Design review of the part shown in the three views and the two pictorial views. Dimensions are in mm from the part's minimum x, y and z. A direction names the side the tool comes from. Coordinates: 2 decimals unless noted, no trailing zeros. Write each loop counter-clockwise with the first axis right and the second up, starting at its lowest first coordinate (ties: lowest second). Pieces come first, ordered by that corner, then holes. Notation, with made-up numbers: (-2.75, -11) - (41.25, -11) arc R22 cw to (41.25, 18) - close; hole circle Ø11 at (32.5, 82.5). An arc over 180 degrees is marked (long way). Return JSON: item names as keys, results as strings. Group by question number.
(1) We need section A-A on x = 4.5. State the section outline as (y, z) points.
(2) We need section C-C on z = 6. State the section outline as (x, y) points.
(3) To check wall thickness, follow L1, parallel to Y at x = 4.5, z = 5; L2, parallel to Y at x = 6, z = 1; L3, parallel to X at y = 5.75, z = 10.75. State the ranges of each line that lie inside material, in increasing order. Write a range as from..to.
(4) Tool access review of the marked faces 4 and 5: name each direction out of +Z, -Z, +X, -X, +Y, -Y from which nothing blocks a thin tool from reaching the whole face with its end or side.
(5) We need section D-D on x = 1.5. State the section outline as (y, z) points.
(6) Draft analysis for pull direction Y (two halves, no side actions). For the marked faces 1, 2 and 3, state which applies: released by +Y, released by -Y, zero draft, split by the parting line, or undercut.
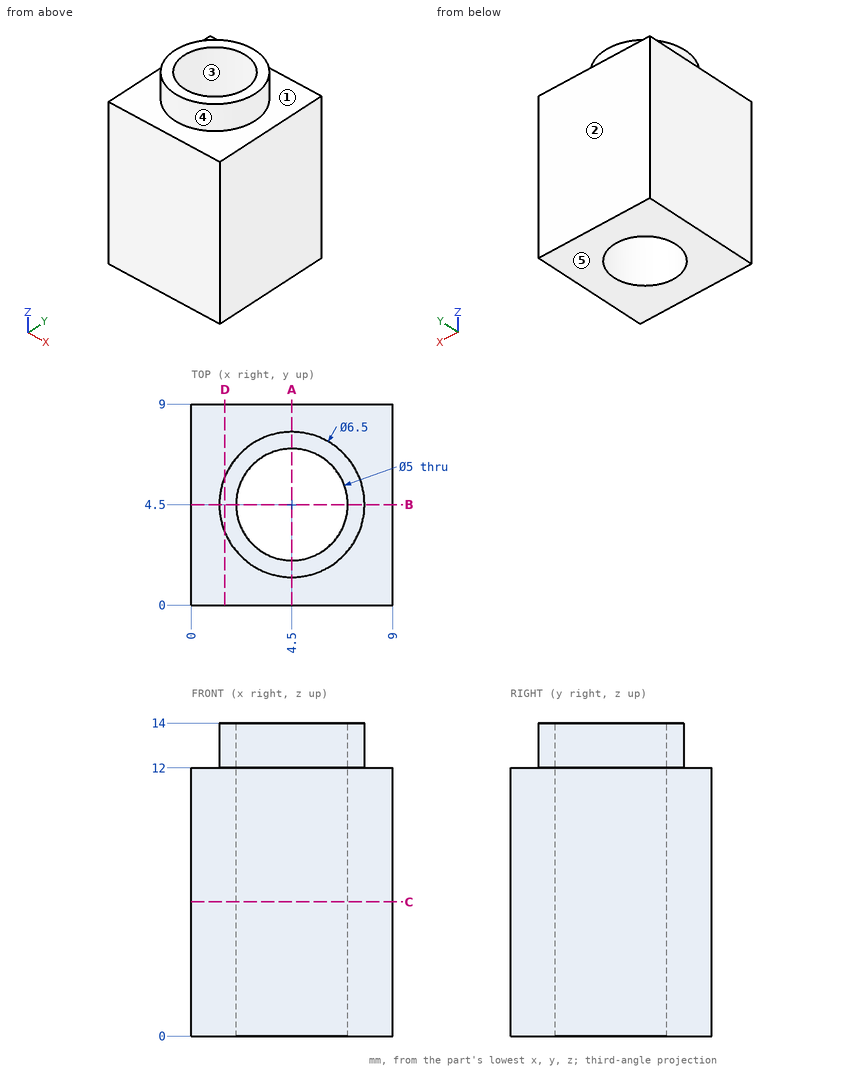
Ans:
{
 "1": {"outline": "(0, 0) - (2, 0) - (2, 14) - (1.25, 14) - (1.25, 12) - (0, 12) - close; (7, 0) - (9, 0) - (9, 12) - (7.75, 12) - (7.75, 14) - (7, 14) - close"},
 "2": {"outline": "(0, 0) - (9, 0) - (9, 9) - (0, 9) - close; hole circle Ø5 at (4.5, 4.5)"},
 "3": {"L1": "0..2, 7..9", "L2": "0..2.5, 6.5..9", "L3": "0..2.33, 6.67..9"},
 "4": {"face 4": "+Z", "face 5": "-Z, +X, -X, +Y, -Y"},
 "5": {"outline": "(0, 0) - (9, 0) - (9, 12) - (5.75, 12) - (5.75, 14) - (3.25, 14) - (3.25, 12) - (0, 12) - close"},
 "6": {"face 1": "zero draft", "face 2": "released by +Y", "face 3": "undercut"}
}
